Autodesk Inventor part; units mm, degrees
ref_plane "YZ Plane" through (0, 0, 0) normal (1, 0, 0) x (0, 1, 0)
ref_plane "XZ Plane" through (0, 0, 0) normal (0, 1, 0) x (-1, 0, 0)
sketch "Sketch1" plane through (0, 0, 0) normal (0, 1, 0) x (-1, 0, 0)
  circle A0 centre (0, 0) radius 10
  dimension "d0" = 20
extrude "Extrusion1" add sketch "Sketch1" along normal blind 26
sketch "Sketch2" plane through (0, 0, 0) normal (0, -1, 0) x (1, 0, 0)
  point P0 (0, 0)
  point P1 (0, 0)
hole "Hole1" at (0, 0, 0) direction (0, 1, 0) diameter 5.5 end through all counterbore diameter 10 counterbore depth 5.5
sketch "Sketch3" plane through (0, 0, 0) normal (1, 0, 0) x (0, 1, 0)
  line L0 (24.5, 10) -> (1.5, 10)
  line L1 (1.5, 10) -> (1.5, 6)
  line L2 (1.5, 6) -> (24.5, 6)
  line L3 (24.5, 6) -> (24.5, 10)
  line L4 (26, -10) -> (26, 10)
  line L5 (-4.4, 0) -> (26.4, 0)
  point P0 (0, 0)
  dimension "d10" = 6
  dimension "d11" = 1.5
  dimension "d12" = 1.5
revolve "Revolution1" cut sketch "Sketch3" angle 360 about axis through (0, -10, 0) along (0, 1, 0)
sketch "Sketch5" plane through (0, 26, 0) normal (0, 1, 0) x (1, 0, 0)
  circle A0 centre (0, 0) radius 2.75
hole "Hole2" at (0, 26, 0) direction (0, -1, 0) diameter 5.5 end through all counterbore diameter 10 counterbore depth 5.5
sketch "Sketch7" plane through (0, 0, 0) normal (1, 0, 0) x (0, 1, 0)
  line L0 (-12.4894, -25.9847) -> (40.6535, -25.9847)
  line L1 (40.6535, -25.9847) -> (40.6535, 26.2362)
  line L2 (40.6535, 26.2362) -> (-12.4894, 26.2362)
  line L3 (-12.4894, 26.2362) -> (-12.4894, -25.9847)
  point P0 (0, 0)
extrude "Extrusion3" cut sketch "Sketch7" against normal blind 15
ref_plane "Work Plane1" through (0, 0, 6) normal (0, 0, 1) x (1, 0, 0)
sketch "Sketch8" plane through (0, 0, 6) normal (0, 0, 1) x (1, 0, 0)
  line L0 (0, 0) -> (10, 0)
  line L1 (0, 1.5) -> (10, 1.5)
  line L2 (0, 0) -> (4, 0)
  line L3 (4, 0) -> (4, 1.5)
  line L4 (4, 1.5) -> (0, 1.5)
  line L5 (0, 1.5) -> (0, 0)
  line L6 (0, 20.5) -> (0, 26)
  line L7 (10, 24.5) -> (0, 24.5)
  line L8 (0, 26) -> (4, 26)
  line L9 (4, 26) -> (4, 24.5)
  line L10 (4, 24.5) -> (0, 24.5)
  line L11 (0, 24.5) -> (0, 26)
  dimension "d26" = 4
extrude "Extrusion4" add sketch "Sketch8" along normal blind 10
properties part number "Test2" material "ABS Plastic"
Read the model definition and answer for the solid it produces. Units are mm, in the model's axes. A direction names the side the tool comes from. Round coordinates to 2 decimals unless told otherwise and drop trailing zeros. Order: outer loops, then holes, each group sorted by start corner. A loop starts at its lowest first (then second) coordinate and runs counter-clockwise, first axis right, second up.
1) For faces 1 (the face through (6, 13, 0)), 2 (the face through (5, 3, 0)), 3 (the face through (5, 23, 0)), 4 (the face through (4, 25, 13)), determine the directions among +Z, -Z, +X, -X, +Y, -Y from which every point of the face is accessible in a straight line to the end or side of a thin tool.
2) The mould has two halves that part along Z. Classify faces 5 (the face through (0, 12, 5)), 6 (the face through (2, 25, 16)), 7 (the face through (3, 20.5, 0)): released by +Z, released by -Z, zero draft, split by the parting line, or undercut.
3) The part is cut by section D-D on y = 15.75. Write down the section's boundary in (x, z), plus the area to 3 significant figures.
4) Straight lines are drawn through the part: L1, parallel to Y at x = 7.25, z = -3.5; L2, parallel to Z at x = 2.5, y = 19.75; L3, parallel to Z at x = 8, y = 1. For each, find the intervals that lie inside material, in ascending order.
5) The part is cut by section B-B on x = 9. Write down the section's boundary in (y, z), plus the area to 3 significant figures.
6) The part is cut by section C-C on z = 0. Write down the section's boundary in (x, y).
7) Flat-ended cylindrical pins translate along their axes: pin 1 (2.5 mm diameter, centred on x = 1.5, z = -1.5, fed in from -Y); pin 2 (2 mm diameter, centred on x = 8, y = 23, fed in from -Z); pin 3 (1.2 mm diameter, centred on y = 1, z = 12.5, fed in from +X); pin 4 (3 mm diameter, centred on y = 18, z = 5, fed in from +X). Find the tip coordinate at first contact, or state that the pin passes through.
8) The part is cut by section A-A on z = 10.25. Write down the section's boundary in (x, y), plus the area to 3 significant figures.
Resolved:
1. face 1: +X
1. face 2: -X, -Y
1. face 3: -X, +Y
1. face 4: +Z, +X, +Y, -Y
2. face 5: zero draft
2. face 6: released by +Z
2. face 7: undercut
3. outline: (0, -6) arc R6 ccw to (0, 6) - (0, 2.75) arc R2.75 cw to (0, -2.75) - close
3. area: 44.7 mm2
4. L1: y = 0 to 1.5, 24.5 to 26
4. L2: z = -5.45 to -1.15, 1.15 to 5.45
4. L3: z = -6 to 6
5. outline: (0, -4.36) - (1.5, -4.36) - (1.5, 4.36) - (0, 4.36) - close; (24.5, -4.36) - (26, -4.36) - (26, 4.36) - (24.5, 4.36) - close
5. area: 26.2 mm2
6. outline: (2.75, 5.5) - (5, 5.5) - (5, 0) - (10, 0) - (10, 1.5) - (6, 1.5) - (6, 24.5) - (10, 24.5) - (10, 26) - (5, 26) - (5, 20.5) - (2.75, 20.5) - close
7. pin 1: stops at y = 5.5
7. pin 2: passes through
7. pin 3: stops at x = 4
7. pin 4: stops at x = 4.87
8. outline: (0, 0) - (4, 0) - (4, 1.5) - (0, 1.5) - close; (0, 24.5) - (4, 24.5) - (4, 26) - (0, 26) - close
8. area: 12.0 mm2
